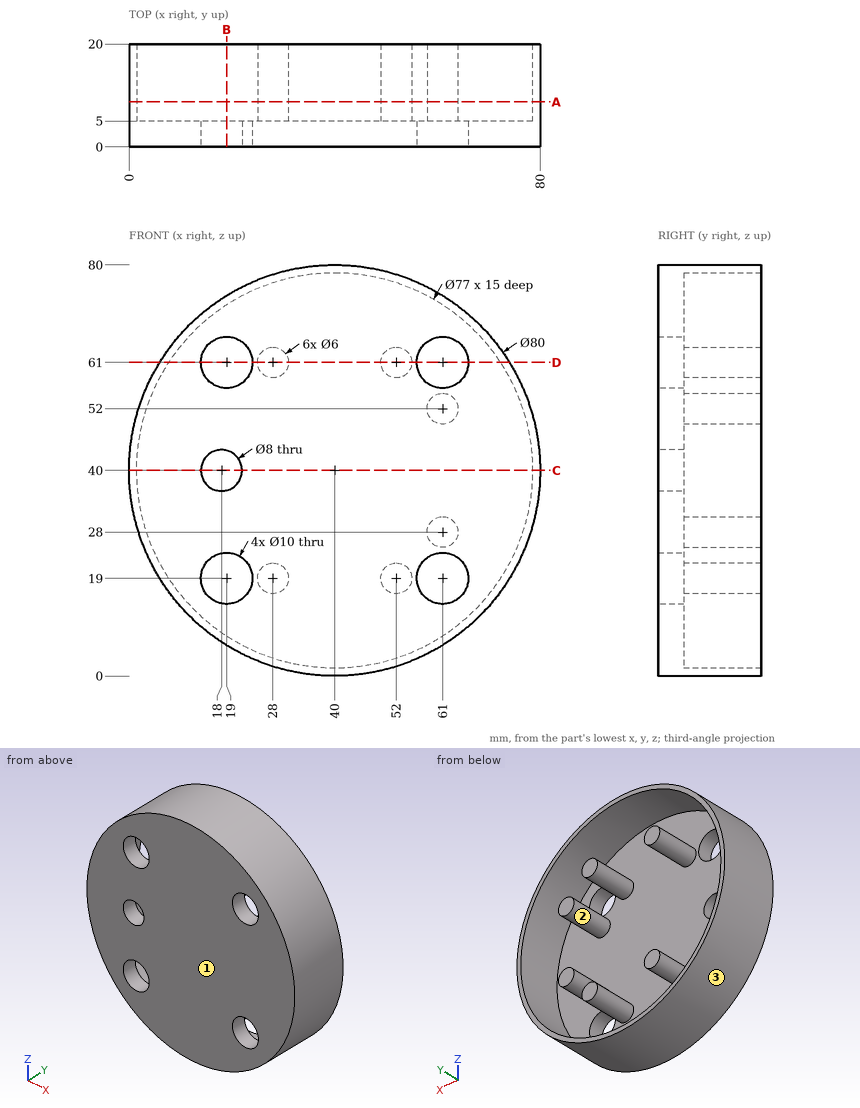
Can you work these out from the drawing? Everything is in mm from the part's minimum corner. Give positions to 0.01 mm unless a question says otherwise; leave off trailing zeros. Order: outer loops, then holes, each group sorted by start corner. A loop starts at its lowest first (then second) coordinate and runs counter-clockwise, first axis right, second up. Notation, with made-up numbers: M 60.5,-13 L 64.5,-13 A20 cw 64.5,22 Z; hole C 31.5,-38 d10. An arc over 180 degrees is marked long. Use a Markdown table: item, result. Add a question column.
1. For pin 1 Ø1 at (x, z) = (43, 22.5) entering from +Y; pin 2 Ø12 at (x, z) = (25.5, 70) entering from +Y; pin 3 Ø5 at (y, z) = (8, 42.5) entering from -X; pin 4 Ø3 at (y, z) = (11.5, 54.5) entering from +X, each with a flat end and sliding along its axis, tell me the tip position at first contact or that it passes through.
2. Suppose I cut it at B-B (x = 19). List the corners of the cut face in (y, z) for me.
3. I need wall thicknesses on probe 1 along X at (y, z) = (12.5, 41); probe 2 along X at (y, z) = (2.6, 61); probe 3 along Z at (x, y) = (30.5, 6). Which ranges of each line are inside material? Lowest first, please. Write a range as from..to.
4. Suppose I cut it at C-C (z = 40). List the corners of the cut face in (x, y) for me, and give its area (3 significant figures).
5. If we mould it in two halves opening along X, with no side actions, what happens to the marked faces 1, 2 and 3? For each: +X half, -X half, draft (parallel to the pull), parting line (faces both ways), or undercut.
6. Suppose I cut it at D-D (z = 61). List the corners of the cut face in (x, y) for me, and give its area (3 significant figures).
7. Suppose I cut it at A-A (y = 8.75). List the corners of the cut face in (x, z) for me, and give its area (3 significant figures).
Results list:
| question | item | result |
|---|---|---|
| 1 | pin 1 | stops at y = 5 |
| 1 | pin 2 | stops at y = 20 |
| 1 | pin 3 | stops at x = 0 |
| 1 | pin 4 | stops at x = 77.83 |
| 2 | outline | M 0,5.96 L 20,5.96 L 20,7.73 L 5,7.73 L 5,14 L 0,14 Z; M 0,24 L 5,24 L 5,36.13 L 0,36.13 Z; M 0,43.87 L 5,43.87 L 5,56 L 0,56 Z; M 0,66 L 5,66 L 5,72.27 L 20,72.27 L 20,74.04 L 0,74.04 Z |
| 3 | probe 1 | x = 0.01..1.51, 78.49..79.99 |
| 3 | probe 2 | x = 5.96..14, 24..56, 66..74.04 |
| 3 | probe 3 | z = 1.14..2.69, 17.34..20.66, 59.34..62.66, 77.31..78.86 |
| 4 | outline | M 0,0 L 14,0 L 14,5 L 1.5,5 L 1.5,20 L 0,20 Z; M 22,0 L 80,0 L 80,20 L 78.5,20 L 78.5,5 L 22,5 Z |
| 4 | area | 405 mm² |
| 5 | face 1 | draft |
| 5 | face 2 | undercut |
| 5 | face 3 | parting line |
| 6 | outline | M 5.96,0 L 14,0 L 14,5 L 7.73,5 L 7.73,20 L 5.96,20 Z; M 24,0 L 56,0 L 56,5 L 55,5 L 55,20 L 49,20 L 49,5 L 31,5 L 31,20 L 25,20 L 25,5 L 24,5 Z; M 66,0 L 74.04,0 L 74.04,20 L 72.27,20 L 72.27,5 L 66,5 Z |
| 6 | area | 474 mm² |
| 7 | outline | C 40,40 d80; C 28,19 d6; C 28,61 d6; C 52,19 d6; C 52,61 d6; C 61,28 d6; C 61,52 d6; hole C 40,40 d77 |
| 7 | area | 540 mm² |
